```python
from build123d import *

# Parameters (mm, degrees)
CYLINDER001_R     = 19.5
CYLINDER001_DEPTH = 30
CYLINDER_R        = 10.3
CYLINDER_DEPTH    = 3
CYLINDER003_R     = 17.9
CYLINDER003_DEPTH = 3


with BuildPart() as cylinder001:
    # Cylinder001 → Cylinder001 (new body)
    with BuildSketch(Plane.XY.offset(60)):
        Circle(CYLINDER001_R)
    extrude(amount=CYLINDER001_DEPTH)


with BuildPart() as fusion:
    # Cylinder → Cylinder (new body)
    with BuildSketch(Plane.XY.offset(57)):
        Circle(CYLINDER_R)
    extrude(amount=CYLINDER_DEPTH)

    # Fusion: union Cylinder001
    add(cylinder001.part)


with BuildPart() as obj1:
    # Cylinder003 → Cylinder003 (new body)
    with BuildSketch(Plane.XY.offset(57)):
        Circle(CYLINDER003_R)
    extrude(amount=CYLINDER003_DEPTH)

    # Fusion001: union Fusion
    add(fusion.part)


solid = obj1.part
```
Check sheet for the modelled part. Datum: model origin and axes. Units: mm. A direction names the side the tool comes from. Coordinates: 2 decimals unless noted, no trailing zeros. Loops run counter-clockwise (first coordinate to the right, second up) from the corner with the lowest first, then second, coordinate; pieces in that order, holes last.
1) Sectioned sample at B-B (y = -10). Record the boundary of the cut face in (x, z), and give its area (3 significant figures).
2) Sectioned sample at C-C (z = 68). Record the boundary of the cut face in (x, y).
3) Gauge pin test, flat ends, axial feed: pin 1 (3 mm diameter, centred on y = -12.5, z = 70, fed in from +X); pin 2 (5 mm diameter, centred on y = 4.5, z = 60.5, fed in from +X); pin 3 (12 mm diameter, centred on x = 4.5, z = 80, fed in from -Y). Record the tip position at first contact, or that the pin passes through.
4) Material ranges on probe 1 along Z at (x, y) = (16, -10); probe 2 along Y at (x, z) = (16, 85.5); probe 3 along Y at (x, z) = (5, 68.5), recorded low to high.
5) Access from +Z, -Z, +X, -X, +Y, -Y to the whole of each face (thin tool, end or side, straight path). Record for faces 1 (the face through (9, -16, 60)), 2 (the face through (0, 0, 90)).
6) Sectioned sample at A-A (x = -14). Record the boundary of the cut face in (y, z).
Check sheet entries:
1. outline: (-16.74, 60) - (-14.85, 60) - (-14.85, 57) - (14.85, 57) - (14.85, 60) - (16.74, 60) - (16.74, 90) - (-16.74, 90) - close
1. area: 1,090 mm2
2. outline: circle Ø39 at (0, 0)
3. pin 1: stops at x = 16.1
3. pin 2: stops at x = 19.4
3. pin 3: stops at y = -19.5
4. probe 1: z = 60 to 90
4. probe 2: y = -11.15 to 11.15
4. probe 3: y = -18.85 to 18.85
5. face 1: -Z
5. face 2: +Z, +X, -X, +Y, -Y
6. outline: (-13.57, 60) - (-11.15, 60) - (-11.15, 57) - (11.15, 57) - (11.15, 60) - (13.57, 60) - (13.57, 90) - (-13.57, 90) - close
